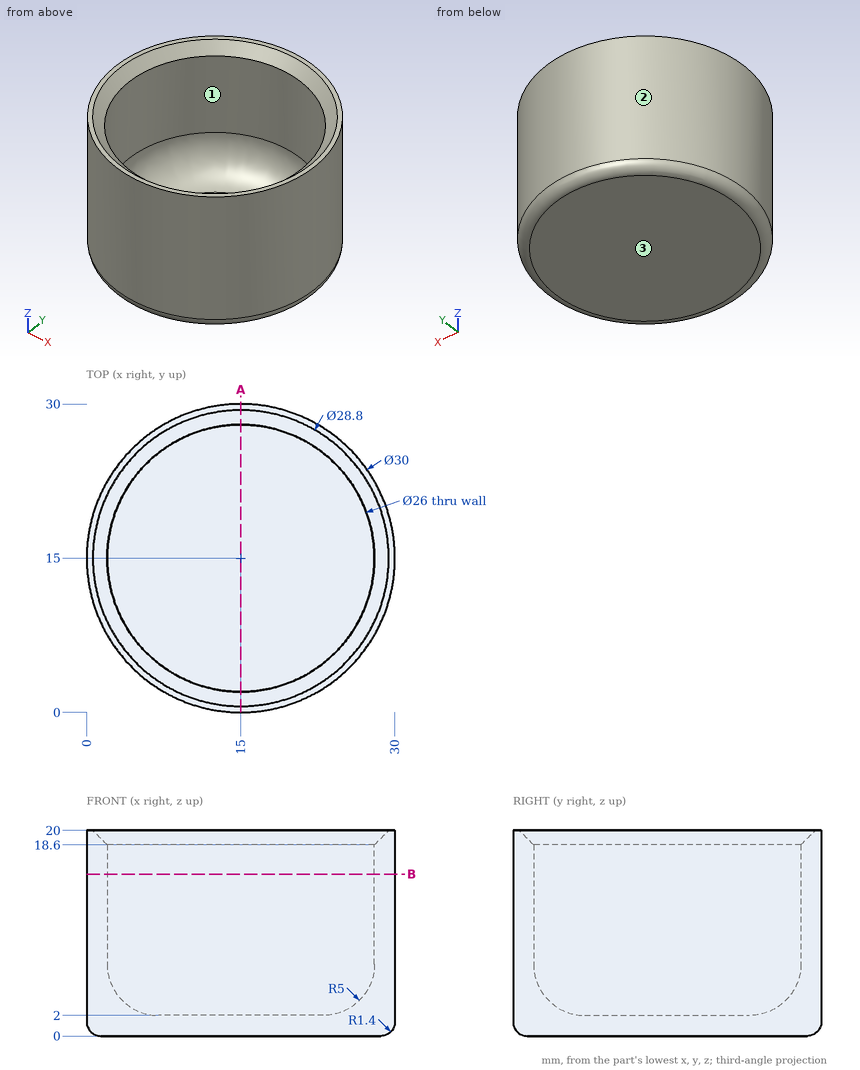
Part print with two shaded views. Sizes in mm from the minimum x, y, z corner. Round coordinates to 2 decimals unless told otherwise and drop trailing zeros. Order: outer loops, then holes, each group sorted by start corner. A loop starts at its lowest first (then second) coordinate and runs counter-clockwise, first axis right, second up. Notation, with made-up numbers: M 88,13.25 L 147,13.25 A17 ccw 147,24.25 Z; hole C 74,33 d11. An arc over 180 degrees is marked long. Put each result on its own line as item: value. Start each with the question number.
1. Two-plate mould, pull along X, no slides. Class the marked faces 1, 2 and 3: +X half, -X half, draft (parallel to the pull), parting line (faces both ways), or undercut.
2. Drop flat-ended pins along their axis: pin 1 (1 mm diameter, centred on y = 17, z = 5, fed in from +X); pin 2 (2 mm diameter, centred on x = 16, z = 7.5, fed in from +Y); pin 3 (5 mm diameter, centred on y = 24.5, z = 14.5, fed in from +X); pin 4 (6 mm diameter, centred on x = 5.5, z = 17.5, fed in from +Y). Give the stop position or say it passes through.
3. Drill centre lines: probe 1 along Y at (x, z) = (15, 15.5); probe 2 along Z at (x, y) = (13.75, 16); probe 3 along Y at (x, z) = (19.25, 7). Where is each one in solid material? Low to high. Write a range as [from, to].
4. Slice it at A-A on x = 15. List the corners of the cut face in (y, z).
5. Slice it at B-B on z = 15.75. List the corners of the cut face in (x, y).
Findings:
1. face 1: undercut
1. face 2: parting line
1. face 3: draft
2. pin 1: x = 29.92
2. pin 2: y = 30
2. pin 3: x = 28.27
2. pin 4: y = 28.52
3. probe 1: [0, 2], [28, 30]
3. probe 2: [0, 2]
3. probe 3: [0.61, 2.71], [27.29, 29.39]
4. outline: M 0,1.4 A1.4 ccw 1.4,0 L 28.6,0 A1.4 ccw 30,1.4 L 30,20 L 29.4,20 L 28,18.6 L 28,7 A5 cw 23,2 L 7,2 A5 cw 2,7 L 2,18.6 L 0.6,20 L 0,20 Z
5. outline: C 15,15 d30; hole C 15,15 d26
